Build history of the part. All positions in model axes, mm. Face numbers are marked on the shaded views. A direction names the side the tool comes from. Give positions to 0.01 mm unless a question says otherwise; leave off trailing zeros. Loops run counter-clockwise (first coordinate to the right, second up) from the corner with the lowest first, then second, coordinate; pieces in that order, holes last. Notation, with made-up numbers: (20.5, 2.25) -> (66.5, 2.25) arc R24 cw to (66.5, 13.25) -> close; hole circle Ø4 at (48.25, 52). An arc over 180 degrees is marked (long way). One line per question, with ' | ' between items. Start each with the question number.
(1) Drill centre lines: L1, parallel to Y at x = 56, z = 5.75; L2, parallel to Y at x = 53.5, z = 2.5; L3, parallel to Z at x = -16, y = -27. Where is each one in solid material? Low to high. Write a range as from..to.
(2) Slice it at A-A, the plane x = -3.5. Write the cut outline in (y, z).
(3) Flat gauge pins, fed straight in: pin 1 Ø1 at (y, z) = (-10, 7.5) entering from -X; pin 2 Ø6 at (x, z) = (61, 11) entering from -Y; pin 3 Ø3 at (x, y) = (34.24, -3.1) entering from -Z; pin 4 Ø6 at (x, y) = (-4, -15.5) entering from +Z. Where does each tip first touch, or does it go through?
(4) Slice it at B-B, the plane z = 18.75. Write the cut outline in (x, y), then the cut area to 3 significant figures.
(5) 3-axis set-ups, long thin cutter, end or side, ignore diameter. For the marked faces 1, 2 and 3: which of +Z, -Z, +X, -X, +Y, -Y reach the whole face in a straight line?
```python
from build123d import *

# Parameters (mm, degrees)
BOSS_EXTRUDE1_DEPTH     = 3
FILLET1_R               = 0.5
BOSS_EXTRUDE3_DEPTH     = 24
FILLET4_R               = 3
FILLET5_R               = 3
FILLET6_R               = 3
SKETCH4_W               = 6
SKETCH4_H               = 4
BOSS_EXTRUDE4_DEPTH     = 6
FILLET7_R               = 2
SKETCH7_W               = 8
SKETCH7_H               = 20
BOSS_EXTRUDE5_DEPTH     = 6
FILLET8_R               = 2
CUT_EXTRUDE1_DEPTH      = 31.137490822
CUT_EXTRUDE1_DEPTH_BACK = 7.874
SKETCH5_R               = 1.5
CUT_EXTRUDE2_DEPTH      = 31.137490822
SKETCH12_R              = 3
SKETCH12_R_2            = 2.5
CUT_EXTRUDE3_DEPTH      = 31.137490822
SKETCH13_R              = 1.5
CUT_EXTRUDE4_DEPTH      = 31.137490822
CIRPATTERN1_COUNT       = 4
SKETCH14_R              = 0.8
CUT_EXTRUDE5_DEPTH      = 31.137490822


with BuildPart() as part:
    # Sketch1 → Boss-Extrude1 (new body)
    with BuildSketch(Plane.XY):
        Polygon((-18.861888764, -42.099818659), (82.138111236, -42.099818659), (82.138111236, -19.099818659), (70.138111236, -19.099818659), (70.138111236, -13.099818659), (82.138111236, -13.099818659), (82.138111236, 6.900181341), (70.138111236, 6.900181341), (70.138111236, 12.900181341), (82.138111236, 12.900181341), (82.138111236, 28.900181341), (54.138111236, 35.900181341), (-18.861888764, 35.900181341), (-27.861888764, 28.900181341), (-33.361888764, 11.900181341), (-33.361888764, -18.099818659), (-27.861888764, -35.099818659), align=None)
    extrude(amount=BOSS_EXTRUDE1_DEPTH)

    # Fillet1
    fillet1_edges = [part.edges().sort_by_distance(p)[0] for p in [
        (-30.611888764, -26.599818659, 0),
        (-33.361888764, -3.099818659, 0),
        (-30.611888764, 20.400181341, 0),
        (-23.361888764, 32.400181341, 0),
        (17.638111236, 35.900181341, 0),
        (68.138111236, 32.400181341, 0),
        (82.138111236, 20.900181341, 0),
        (76.138111236, 12.900181341, 0),
        (70.138111236, 9.900181341, 0),
        (76.138111236, 6.900181341, 0),
        (82.138111236, -3.099818659, 0),
        (76.138111236, -13.099818659, 0),
        (70.138111236, -16.099818659, 0),
        (76.138111236, -19.099818659, 0),
        (82.138111236, -30.599818659, 0),
        (31.638111236, -42.099818659, 0),
        (-23.361888764, -38.599818659, 0),
    ]]
    fillet(fillet1_edges, radius=FILLET1_R)

    # Sketch2 → Boss-Extrude3 (add)
    with BuildSketch(Plane.XY.offset(3)):
        Polygon((63.638111236, -19.099818659), (46.638111236, -19.099818659), (46.638111236, 12.900181341), (63.638111236, 12.900181341), (63.638111236, 4.100181341), (52.638111236, 4.100181341), (52.638111236, -10.299818659), (63.638111236, -10.299818659), align=None)
    extrude(amount=BOSS_EXTRUDE3_DEPTH)

    # Fillet4
    fillet4_edges = [part.edges().sort_by_distance(p)[0] for p in [
        (46.638111236, -3.099818659, 27),
    ]]
    fillet(fillet4_edges, radius=FILLET4_R)

    # Fillet5
    fillet5_edges = [part.edges().sort_by_distance(p)[0] for p in [
        (63.638111236, 8.500181341, 27),
        (63.638111236, -14.699818659, 27),
    ]]
    fillet(fillet5_edges, radius=FILLET5_R)

    # Fillet6
    fillet6_edges = [part.edges().sort_by_distance(p)[0] for p in [
        (63.638111236, -14.699818659, 3),
        (63.638111236, 8.500181341, 3),
    ]]
    fillet(fillet6_edges, radius=FILLET6_R)

    # Sketch4 → Boss-Extrude4 (add)
    with BuildSketch(Plane.XY.offset(3)):
        with Locations((79.138111236, -21.099818659)):
            Rectangle(SKETCH4_W, SKETCH4_H)
    extrude(amount=BOSS_EXTRUDE4_DEPTH)

    # Fillet7
    fillet7_edges = [part.edges().sort_by_distance(p)[0] for p in [
        (82.138111236, -21.099818659, 9),
        (76.138111236, -21.099818659, 9),
    ]]
    fillet(fillet7_edges, radius=FILLET7_R)

    # Sketch7 → Boss-Extrude5 (add)
    with BuildSketch(Plane.XY.offset(3)):
        with Locations((78.138111236, -3.099818659)):
            Rectangle(SKETCH7_W, SKETCH7_H)
    extrude(amount=BOSS_EXTRUDE5_DEPTH)

    # Fillet8
    fillet8_edges = [part.edges().sort_by_distance(p)[0] for p in [
        (82.138111236, -3.099818659, 9),
        (74.138111236, -3.099818659, 9),
    ]]
    fillet(fillet8_edges, radius=FILLET8_R)

    # Sketch5 → Cut-Extrude1 (cut, two sides: drawn at the far end of the back side and taken through both)
    with BuildSketch(Plane(origin=(0, -19.099818659, 0), x_dir=(1, 0, 0), z_dir=(0, 1, 0)).offset(-CUT_EXTRUDE1_DEPTH_BACK)):
        with Locations(Location((79.138111236, -6, 0), (0, 0, 90))):
            Circle(SKETCH5_R)
    extrude(amount=CUT_EXTRUDE1_DEPTH + CUT_EXTRUDE1_DEPTH_BACK, mode=Mode.SUBTRACT)

    # Sketch11 → Cut-Extrude2 (cut)
    with BuildSketch(Plane(origin=(52.638111236, 0, 0), x_dir=(0, 0, -1), z_dir=(1, 0, 0))):
        Polygon((-3, 4.100181341), (-15, 4.100181341), (-15, -10.382699653), (-3, -10.299818659), align=None)
    extrude(amount=-CUT_EXTRUDE2_DEPTH, mode=Mode.SUBTRACT)

    # Sketch12 → Cut-Extrude3 (cut)
    with BuildSketch(Plane.XY.offset(3)):
        with Locations((56.638111236, -3.099818659)):
            Circle(SKETCH12_R)
        with Locations((34.238111236, -3.099818659)):
            Circle(SKETCH12_R_2)
    extrude(amount=-CUT_EXTRUDE3_DEPTH, mode=Mode.SUBTRACT)

    # Sketch13 → Cut-Extrude4 (cut)
    with BuildSketch(Plane.XY.offset(3)):
        with Locations((60.880751923, 1.142822028)):
            Circle(SKETCH13_R)
    cut_extrude4 = extrude(amount=-CUT_EXTRUDE4_DEPTH, mode=Mode.SUBTRACT)

    # CirPattern1: Cut-Extrude4 ×4 about axis
    cirpattern1_axis = Axis((56.638111236, -3.099818659, 0), (0, 0, 1))
    for i in range(1, CIRPATTERN1_COUNT):
        add(cut_extrude4.rotate(cirpattern1_axis, i * 360 / CIRPATTERN1_COUNT), mode=Mode.SUBTRACT)

    # Sketch14 → Cut-Extrude5 (cut)
    with BuildSketch(Plane.XY.offset(3)):
        with Locations((34.238111236, 1.400181341)):
            Circle(SKETCH14_R)
        with Locations((34.238111236, -7.599818659)):
            Circle(SKETCH14_R)
    extrude(amount=-CUT_EXTRUDE5_DEPTH, mode=Mode.SUBTRACT)


solid = part.part
```
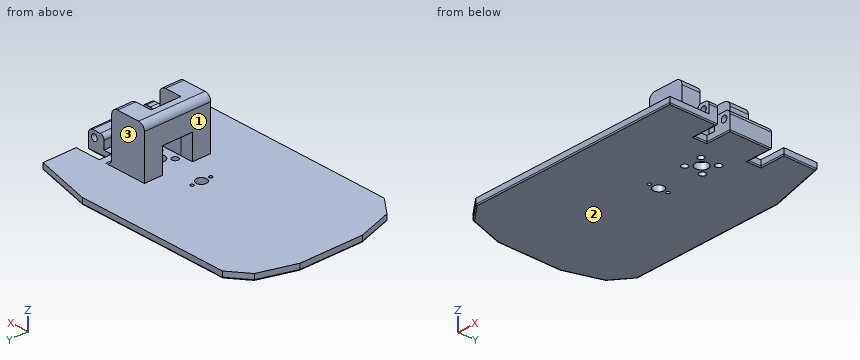
Final values:
1) L1: -19.1..-10.3, 4.1..12.9 | L2: -42.1..-8.36, -6.33..0.13, 2.16..35.9 | L3: 0..3
2) outline: (-42.1, 0.5) arc R0.5 ccw to (-41.6, 0) -> (35.4, 0) arc R0.5 ccw to (35.9, 0.5) -> (35.9, 3) -> (-42.1, 3) -> close
3) pin 1: x = 46.64 | pin 2: y = -19.1 | pin 3: through | pin 4: z = 3
4) outline: (46.64, -19.1) -> (63.64, -19.1) -> (63.64, -10.3) -> (52.64, -10.3) -> (52.64, 4.1) -> (63.64, 4.1) -> (63.64, 12.9) -> (46.64, 12.9) -> close | area: 386 mm2
5) face 1: +Z, -X, +Y, -Y | face 2: -Z, +X, -X, +Y, -Y | face 3: +Z, +X, -X, +Y
